from build123d import *

# Parameters (mm, degrees)
SKETCH036_W     = 126
SKETCH036_H     = 140
PAD017_DEPTH    = 43
THICKNESS_T     = -3
CHAMFER017_SIZE = 2
SKETCH037_R     = 2.25
POCKET018_DEPTH = 126.001
CHAMFER018_SIZE = 1
SKETCH038_R     = 3.3
POCKET019_DEPTH = 5
CHAMFER019_SIZE = 0.3
SKETCH039_R     = 2.3
POCKET020_DEPTH = 3.001
CHAMFER020_SIZE = 0.25


with BuildPart() as part:
    # Sketch036 → Pad017 (new body)
    with BuildSketch(Plane.XY):
        Rectangle(SKETCH036_W, SKETCH036_H)
    extrude(amount=PAD017_DEPTH)

    # Thickness
    thickness_openings = [part.faces().sort_by_distance(p)[0] for p in [
        (0, 0, 0),
    ]]
    offset(amount=THICKNESS_T, openings=thickness_openings, kind=Kind.INTERSECTION)

    # Chamfer017
    chamfer017_edges = [part.edges().sort_by_distance(p)[0] for p in [
        (-60, -67, 20),
        (-60, 0, 40),
        (0, -67, 40),
        (-60, 67, 20),
        (0, 67, 40),
        (60, 67, 20),
        (60, 0, 40),
        (60, -67, 20),
    ]]
    chamfer(chamfer017_edges, length=CHAMFER017_SIZE)

    # Sketch037 (on Face13 of Chamfer017) → Pocket018 (cut, through all)
    with BuildSketch(Plane(origin=(-63, 0, 0), x_dir=(0, -1, 0), z_dir=(-1, 0, 0))):
        with Locations((-45, 8)):
            Circle(SKETCH037_R)
        with Locations((45, 8)):
            Circle(SKETCH037_R)
    extrude(amount=-POCKET018_DEPTH, mode=Mode.SUBTRACT)

    # Chamfer018
    chamfer018_edges = [part.edges().sort_by_distance(p)[0] for p in [
        (-63, -70, 21.5),
        (-63, 0, 0),
        (-63, 0, 43),
        (-63, 70, 21.5),
        (-63, -42.75, 8),
        (-63, 47.25, 8),
        (63, -70, 21.5),
        (0, -70, 0),
        (0, -70, 43),
        (63, 70, 21.5),
        (63, 0, 0),
        (63, 0, 43),
        (63, -42.75, 8),
        (63, 47.25, 8),
        (0, 70, 0),
        (0, 70, 43),
    ]]
    chamfer(chamfer018_edges, length=CHAMFER018_SIZE)

    # Sketch038 (on Face18 of Chamfer018) → Pocket019 (cut)
    with BuildSketch(Plane.XZ.offset(70)):
        with Locations((-20, 21.5)):
            Circle(SKETCH038_R)
        with Locations((20, 21.5)):
            Circle(SKETCH038_R)
    extrude(amount=-POCKET019_DEPTH, mode=Mode.SUBTRACT)

    # Chamfer019
    chamfer019_edges = [part.edges().sort_by_distance(p)[0] for p in [
        (-23.3, -70, 21.5),
        (-16.7, -68.5, 21.5),
        (-23.3, -67, 21.5),
        (16.7, -70, 21.5),
        (23.3, -68.5, 21.5),
        (16.7, -67, 21.5),
    ]]
    chamfer(chamfer019_edges, length=CHAMFER019_SIZE)

    # Sketch039 (on Face20 of Chamfer019) → Pocket020 (cut, through all)
    with BuildSketch(Plane(origin=(0, 0, 40), x_dir=(1, 0, 0), z_dir=(0, 0, -1))):
        with Locations((0, 48)):
            Circle(SKETCH039_R)
        with Locations((0, -48)):
            Circle(SKETCH039_R)
    extrude(amount=-POCKET020_DEPTH, mode=Mode.SUBTRACT)

    # Chamfer020
    chamfer020_edges = [part.edges().sort_by_distance(p)[0] for p in [
        (-2.3, -48, 40),
        (2.3, -48, 41.5),
        (-2.3, -48, 43),
        (-2.3, 48, 40),
        (2.3, 48, 41.5),
        (-2.3, 48, 43),
    ]]
    chamfer(chamfer020_edges, length=CHAMFER020_SIZE)


solid = part.part
The model under review builds one solid part; all positions refer to its coordinate system, in mm. A direction names the side the tool comes from. Round coordinates to 2 decimals unless told otherwise and drop trailing zeros. Order: outer loops, then holes, each group sorted by start corner. A loop starts at its lowest first (then second) coordinate and runs counter-clockwise, first axis right, second up. Notation, with made-up numbers: (42.25, 0) -> (53.25, 0) arc R32 cw to (53.25, 35) -> close; hole circle Ø8 at (-3.75, 18.25). An arc over 180 degrees is marked (long way). Return JSON: item names as keys, results as strings.
1. For L1, parallel to Y at x = 0, z = 41.85; L2, parallel to Z at x = -61, y = 45; L3, parallel to X at y = 30, z = 15, list the stretches that pass through material, from the lowest coordinate up. Write a range as [from, to].
Answer block:
{"L1": "y = [-70, -50.3], [-45.7, 45.7], [50.3, 70]", "L2": "z = [0, 5.75], [10.25, 43]", "L3": "x = [-63, -60], [60, 63]"}
2. The part is to be moulded in two halves that separate along Y. For faces 3 (the face through (-1, 70, 21)), 4 (the face through (-18.48, -68.52, 18.57)), 5 (the face through (-0.499, -45.755, 41.482)), say which applies: +Y half, -Y half, draft (parallel to the pull), parting line (faces both ways), or undercut.
Answer block:
{"face 3": "+Y half", "face 4": "draft", "face 5": "undercut"}
3. Insertion check: P1, Ø5.5, axis at x = 0, y = -48, coming from the -Z side; P2, Ø5, axis at y = 45, z = 8, coming from the +X side; P3, Ø6, axis at x = -20, z = 21.5, coming from the -Y side. Each pin has a flat end and moves straight along its axis. Give the tip position at first contact, or say it passes through.
Answer block:
{"P1": "stops at z = 40", "P2": "stops at x = 62.25", "P3": "stops at y = 67"}
4. Take a section at C-C (z = 3). Write out the cut boundary in (x, y), then the cut area to 3 significant figures.
Answer block:
{"outline": "(-63, -69) -> (-62, -70) -> (62, -70) -> (63, -69) -> (63, 69) -> (62, 70) -> (-62, 70) -> (-63, 69) -> close; hole (-60, -65) -> (-58, -67) -> (58, -67) -> (60, -65) -> (60, 65) -> (58, 67) -> (-58, 67) -> (-60, 65) -> close", "area": "1,570 mm²"}
5. Take a section at A-A (x = 20). Write out the cut boundary in (y, z).
Answer block:
{"outline": "(-70, 1) -> (-69, 0) -> (-67, 0) -> (-67, 17.9) -> (-67.3, 18.2) -> (-69.7, 18.2) -> (-70, 17.9) -> close; (-70, 25.1) -> (-69.7, 24.8) -> (-67.3, 24.8) -> (-67, 25.1) -> (-67, 38) -> (-65, 40) -> (65, 40) -> (67, 38) -> (67, 0) -> (69, 0) -> (70, 1) -> (70, 42) -> (69, 43) -> (-69, 43) -> (-70, 42) -> close"}
6. For faces 1 (the face through (-1, 1, 43)), 2 (the face through (-60, -1, 19)), list the 3-axis set-ups (+Z, -Z, +X, -X, +Y, -Y) from which the entire face can be reached by the end or side of a thin tool; tool diameter is ignored.
Answer block:
{"face 1": "+Z, +X, -X, +Y, -Y", "face 2": "-Z"}
7. Take a section at D-D (y = -35.5). Write out the cut boundary in (x, z).
Answer block:
{"outline": "(-63, 1) -> (-62, 0) -> (-60, 0) -> (-60, 38) -> (-58, 40) -> (58, 40) -> (60, 38) -> (60, 0) -> (62, 0) -> (63, 1) -> (63, 42) -> (62, 43) -> (-62, 43) -> (-63, 42) -> close"}
